from build123d import *

# Parameters (mm, degrees)
F1_DEPTH = 508
F2_R     = 12.7
F2_R_2   = 6.35
F3_DEPTH = 7.62
F4_DEPTH = 15.24
F6_DEPTH = 3.302


with BuildPart() as f1:
    # F0 (on Top) → F1 (new body)
    with BuildSketch(Plane.XY):
        Polygon((-16.002, 32.004), (-16.002, 0), (0, 0), (16.002, 0), (16.002, 32.004), (6.35, 32.004), (6.35, 28.702), (12.7, 28.702), (12.7, 3.302), (0, 3.302), (-12.7, 3.302), (-12.7, 28.702), (-6.35, 28.702), (-6.35, 32.004), align=None)
    extrude(amount=F1_DEPTH)

    # F2 (on face) → F3 (join)
    with BuildSketch(Plane.XZ):
        with Locations((0, 491.49)):
            Circle(F2_R)
        with Locations((0, 491.49)):
            Circle(F2_R_2, mode=Mode.SUBTRACT)
        with Locations((0, 16.51)):
            Circle(F2_R)
    extrude(amount=F3_DEPTH)

    # F4 (add): a face of the model
    f4_faces = [f1.faces().sort_by_distance(p)[0] for p in [
        (0, 0, 491.49),
    ]]
    extrude(f4_faces, amount=F4_DEPTH)

    # F5 (on face) → F6 (cut, through all)
    with BuildSketch(Plane.XZ):
        with BuildLine():
            Line((-6.35, 469.9), (-6.35, 38.1))
            ThreePointArc((-6.35, 38.1), (0, 31.75), (6.35, 38.1))
            Line((6.35, 38.1), (6.35, 469.9))
            ThreePointArc((6.35, 469.9), (0, 476.25), (-6.35, 469.9))
        make_face()
    extrude(amount=-F6_DEPTH, mode=Mode.SUBTRACT)


solid = f1.part
Read the model definition and answer for the solid it produces. Units are mm, in the model's axes. A direction names the side the tool comes from. Give positions to 0.01 mm unless a question says otherwise; leave off trailing zeros. Write each loop counter-clockwise with the first axis right and the second up, starting at its lowest first coordinate (ties: lowest second). Pieces come first, ordered by that corner, then holes. Notation, with made-up numbers: (-10.75, 14.25) - (5.25, 14.25) arc R19 ccw to (5.25, 50.25) - close; hole circle Ø1 at (13, 47.25). An arc over 180 degrees is marked (long way). Use CSV: the item, a comma, the result in double quotes. Start each with the question number.
(1) Given P1, Ø12.5, axis at x = -4, z = 22.5, coming from the -Y side; P2, Ø12, axis at x = -7, y = -10, coming from the -Z side; P3, Ø3, axis at x = -10.5, z = 185.5, coming from the -Y side; P4, Ø2, axis at x = 10, y = -10.5, coming from the +Z side, each flat-ended and moving along its own axis, determine where each tip first touches the part or whether it passes through.
(2) For faces 5 (the flat face through (-8, 3.302, 250)), 6 (the flat face through (0, -7.62, 17)), 7 (the cylindrical face through (-2.75, -3.76, 4.11)), determine the directions among +Z, -Z, +X, -X, +Y, -Y from which every point of the face is accessible in a straight line to the end or side of a thin tool.
(3) Find section D-D (x = 1). Give the vertices of the cut face in (y, z), plus the area to 3 significant figures.
(4) Find section A-A (y = 9). Give the vertices of the cut face in (x, z).
(5) Consider line 1 along Y through (x, z) = (11, 230); line 2 along X through (y, z) = (19.5, 50); line 3 along X through (y, z) = (2.5, 377). Determine where each line is inside the solid, lowest interval first.
(6) Find section C-C (z = 16.51). Give the vertices of the cut face in (x, y), plus the area to 3 significant figures.
(7) Find section B-B (z = 301). Give the vertices of the cut face in (x, y).
(8) Determine the mould class of faces 1 (the flat face through (12.7, 16, 250)), 2 (the flat face through (-12.7, 16, 250)), 3 (the flat face through (0, -15.24, 491)), 4 (the flat face through (0, 3, 508)) for opening direction Y: +Y half, -Y half, draft (parallel to the pull), parting line (faces both ways), or undercut.
Findings below:
1,P1,"y = -7.62"
1,P2,"z = 3.9"
1,P3,"y = 0"
1,P4,"through"
2,face 5,"+Z, -Z"
2,face 6,"-Z, +X, -X, -Y"
2,face 7,"-Y"
3,outline,"(-15.24, 485.22) - (-7.62, 485.22) - (-7.62, 478.83) - (0, 478.83) - (0, 476.17) - (3.3, 476.17) - (3.3, 508) - (0, 508) - (0, 504.15) - (-7.62, 504.15) - (-7.62, 497.76) - (-15.24, 497.76) - close; (-7.62, 3.85) - (0, 3.85) - (0, 0) - (3.3, 0) - (3.3, 31.83) - (0, 31.83) - (0, 29.17) - (-7.62, 29.17) - close"
3,area,"692 mm2"
4,outline,"(-16, 0) - (-12.7, 0) - (-12.7, 508) - (-16, 508) - close; (12.7, 0) - (16, 0) - (16, 508) - (12.7, 508) - close"
5,line 1,"0 to 3.3, 28.7 to 32"
5,line 2,"-16 to -12.7, 12.7 to 16"
5,line 3,"-16 to -6.35, 6.35 to 16"
6,outline,"(-16, 0) - (-12.7, 0) - (-12.7, -7.62) - (12.7, -7.62) - (12.7, 0) - (16, 0) - (16, 32) - (6.35, 32) - (6.35, 28.7) - (12.7, 28.7) - (12.7, 3.3) - (-12.7, 3.3) - (-12.7, 28.7) - (-6.35, 28.7) - (-6.35, 32) - (-16, 32) - close"
6,area,"531 mm2"
7,outline,"(-16, 0) - (-6.35, 0) - (-6.35, 3.3) - (-12.7, 3.3) - (-12.7, 28.7) - (-6.35, 28.7) - (-6.35, 32) - (-16, 32) - close; (6.35, 0) - (16, 0) - (16, 32) - (6.35, 32) - (6.35, 28.7) - (12.7, 28.7) - (12.7, 3.3) - (6.35, 3.3) - close"
8,face 1,"undercut"
8,face 2,"undercut"
8,face 3,"-Y half"
8,face 4,"draft"
